Part model, mm, in its own coordinate system. Coordinates: 2 decimals unless noted, no trailing zeros. Order: outer loops, then holes, each group sorted by start corner. A loop starts at its lowest first (then second) coordinate and runs counter-clockwise, first axis right, second up.
```python
from build123d import *

# Parameters (mm, degrees)
F1_DEPTH = 6


with BuildPart() as f1:
    # F0 (on Top) → F1 (new body)
    with BuildSketch(Plane.XY):
        with BuildLine():
            ThreePointArc((-5.640001, 11.753323), (-7.442462, 7.416732), (-11.789711, 5.640129))
            Line((-11.789711, 5.640129), (-199.455415, 6.859855))
            ThreePointArc((-199.455415, 6.859855), (-206.36, 0), (-199.455415, -6.859855))
            Line((-199.455415, -6.859855), (-11.789711, -5.640129))
            ThreePointArc((-11.789711, -5.640129), (-7.415726, -7.443473), (-5.64051, -11.828949))
            Line((-5.64051, -11.828949), (-7.489375, -154.903219))
            ThreePointArc((-7.489375, -154.903219), (0, -162.49), (7.489375, -154.903219))
            Line((7.489375, -154.903219), (5.64051, -11.828949))
            ThreePointArc((5.64051, -11.828949), (7.415726, -7.443473), (11.789711, -5.640129))
            Line((11.789711, -5.640129), (220.7, -6.859855))
            ThreePointArc((220.7, -6.859855), (227.604585, 0), (220.7, 6.859855))
            Line((220.7, 6.859855), (11.789711, 5.640129))
            ThreePointArc((11.789711, 5.640129), (7.442462, 7.416732), (5.640001, 11.753323))
            Line((5.640001, 11.753323), (5.75, 214))
            Line((5.75, 214), (4.37, 214))
            Line((4.37, 214), (4.260001, 11.754074))
            ThreePointArc((4.260001, 11.754074), (6.469564, 6.438023), (11.79868, 4.260158))
            Line((11.79868, 4.260158), (220.708969, 5.479884))
            ThreePointArc((220.708969, 5.479884), (226.224585, 0), (220.708969, -5.479884))
            Line((220.708969, -5.479884), (11.79868, -4.260158))
            ThreePointArc((11.79868, -4.260158), (6.43679, -6.470805), (4.260625, -11.846781))
            Line((4.260625, -11.846781), (6.10949, -154.921051))
            ThreePointArc((6.10949, -154.921051), (0, -161.11), (-6.10949, -154.921051))
            Line((-6.10949, -154.921051), (-4.260625, -11.846781))
            ThreePointArc((-4.260625, -11.846781), (-6.43679, -6.470805), (-11.79868, -4.260158))
            Line((-11.79868, -4.260158), (-199.464384, -5.479884))
            ThreePointArc((-199.464384, -5.479884), (-204.98, 0), (-199.464384, 5.479884))
            Line((-199.464384, 5.479884), (-11.79868, 4.260158))
            ThreePointArc((-11.79868, 4.260158), (-6.469564, 6.438023), (-4.260001, 11.754074))
            Line((-4.260001, 11.754074), (-4.37, 214))
            Line((-4.37, 214), (-5.75, 214))
            Line((-5.75, 214), (-5.640001, 11.753323))
        make_face()
    extrude(amount=F1_DEPTH)


solid = f1.part
```
(1) Slice it at C-C, the plane x = -40.5. Give the cut face in (y, z), then the cut area to 3 significant figures.
(2) Drop flat-ended pins along their axis: pin 1 (1 mm diameter, centred on x = -38, z = 5.5, fed in from -Y); pin 2 (2 mm diameter, centred on y = 16, z = 1, fed in from -X); pin 3 (3 mm diameter, centred on x = -116, z = 4, fed in from -Y). Give the stop position or say it passes through.
(3) Slice it at B-B, the plane y = 167.5. Give the cut face in (x, z).
(4) Probe line 1 (Y direction, x = 32.5, z = 4.3); line 2 (X direction, y = 28, z = 0.85); line 3 (X direction, y = -102, z = 0.55). List the from-to ranges inside material, lowest first.
Here are the results:
1. outline: (-5.83, 0) - (-4.45, 0) - (-4.45, 6) - (-5.83, 6) - close; (4.45, 0) - (5.83, 0) - (5.83, 6) - (4.45, 6) - close
1. area: 16.6 mm2
2. pin 1: stops at y = -5.81
2. pin 2: stops at x = -5.64
2. pin 3: stops at y = -6.33
3. outline: (-5.72, 0) - (-4.34, 0) - (-4.34, 6) - (-5.72, 6) - close; (4.34, 0) - (5.72, 0) - (5.72, 6) - (4.34, 6) - close
4. line 1: y = -5.76 to -4.38, 4.38 to 5.76
4. line 2: x = -5.65 to -4.27, 4.27 to 5.65
4. line 3: x = -6.81 to -5.43, 5.43 to 6.81
